Build history of the part. All positions in model axes, mm. Round coordinates to 2 decimals unless told otherwise and drop trailing zeros. Order: outer loops, then holes, each group sorted by start corner. A loop starts at its lowest first (then second) coordinate and runs counter-clockwise, first axis right, second up. Notation, with made-up numbers: (-37, 46.5) -> (4, 46.5) arc R10 cw to (4, 52.5) -> close; hole circle Ø6 at (5.5, -38). An arc over 180 degrees is marked (long way). Use a Markdown table: item, result. Add a question column.
Item 1: Two-plate mould, pull along X, no slides. Class faces 1 (the face through (0, 0, 0)), 2 (the face through (-1, -5.08, 1)), 3 (the face through (-11.012, -55.311, -49.592)): released by +X, released by -X, zero draft, split by the parting line, or undercut.
Item 2: Probe L1, parallel to Z at x = 0, y = -62.5; L2, parallel to X at y = -53.5, z = 6; L3, parallel to X at y = -19.5, z = -19. List the from-to ranges inside material, lowest first.
Item 3: Pin check, flat tips, straight feed: pin 1 (5 mm diameter, centred on y = -19, z = -4.5, fed in from +X); pin 2 (4 mm diameter, centred on x = 34, z = 17.5, fed in from +Y); pin 3 (1.5 mm diameter, centred on x = 5, y = -35, fed in from -Z). Stop position of each tip, or through.
Item 4: Slice it at A-A, the plane y = -44.5. Give the cut face in (x, z), plus the area to 3 significant figures.
from build123d import *

# Parameters (mm, degrees)
F0_R     = 50.8
F1_DEPTH = 101.6
F2_T     = -5.08
F3_R     = 15.24
F4_R     = 5.07999


# Not quite as in the source:
# - a fillet or chamfer is up to 0.001 mm smaller than in the source, because OpenCascade refuses the exact size


with BuildPart() as f1:
    # F0 (on Front) → F1 (new body)
    with BuildSketch(Plane.XZ):
        Circle(F0_R)
    extrude(amount=F1_DEPTH)

    # F2
    f2_openings = [f1.faces().sort_by_distance(p)[0] for p in [
        (0, -101.6, 0),
    ]]
    offset(amount=F2_T, openings=f2_openings)

    # F3
    f3_edges = [f1.edges().sort_by_distance(p)[0] for p in [
        (-50.8, 0, 0),
    ]]
    fillet(f3_edges, radius=F3_R)

    # F4 (radius 5.08 in the source; OpenCascade refuses exactly that, so slightly less here)
    f4_edges = [f1.edges().sort_by_distance(p)[0] for p in [
        (-50.8, -101.6, 0),
    ]]
    fillet(f4_edges, radius=F4_R)


solid = f1.part
Check sheet entries:
| question | item | result |
|---|---|---|
| 1 | face 1 | zero draft |
| 1 | face 2 | undercut |
| 1 | face 3 | split by the parting line |
| 2 | L1 | -50.8 to -45.72, 45.72 to 50.8 |
| 2 | L2 | -50.44 to -45.32, 45.32 to 50.44 |
| 2 | L3 | -47.11 to -41.59, 41.59 to 47.11 |
| 3 | pin 1 | x = 50.76 |
| 3 | pin 2 | y = -0.02 |
| 3 | pin 3 | z = -50.62 |
| 4 | outline | circle Ø101.6 at (0, 0); hole circle Ø91.44 at (0, 0) |
| 4 | area | 1,540 mm2 |
